```python
from build123d import *

# Parameters (mm, degrees)
F0_W     = 75
F0_H     = 75
F1_DEPTH = 75
F2_W     = 25
F2_H     = 25
F3_DEPTH = 25
F4_W     = 25
F4_H     = 25
F5_DEPTH = 25


with BuildPart() as f1:
    # F0 (on Top) → F1 (new body)
    with BuildSketch(Plane.XY):
        with Locations((-11.791817, -4.223716)):
            Rectangle(F0_W, F0_H)
    extrude(amount=F1_DEPTH)

    # F2 (on face) → F3 (cut)
    with BuildSketch(Plane(origin=(0, 0, 0), x_dir=(1, 0, 0), z_dir=(0, 0, -1))):
        with Locations((-36.791817, 29.223716)):
            Rectangle(F2_W, F2_H)
        with Locations((-36.791817, -20.776284)):
            Rectangle(F2_W, F2_H)
        with Locations((13.208183, 29.223716)):
            Rectangle(F2_W, F2_H)
        with Locations((13.208183, -20.776284)):
            Rectangle(F2_W, F2_H)
    extrude(amount=-F3_DEPTH, mode=Mode.SUBTRACT)

    # F4 (on face) → F5 (cut)
    with BuildSketch(Plane.XY.offset(75)):
        with Locations((-36.791817, 20.776284)):
            Rectangle(F4_W, F4_H)
        with Locations((13.208183, 20.776284)):
            Rectangle(F4_W, F4_H)
        with Locations((-36.791817, -29.223716)):
            Rectangle(F4_W, F4_H)
        with Locations((13.208183, -29.223716)):
            Rectangle(F4_W, F4_H)
    extrude(amount=-F5_DEPTH, mode=Mode.SUBTRACT)


solid = f1.part
```
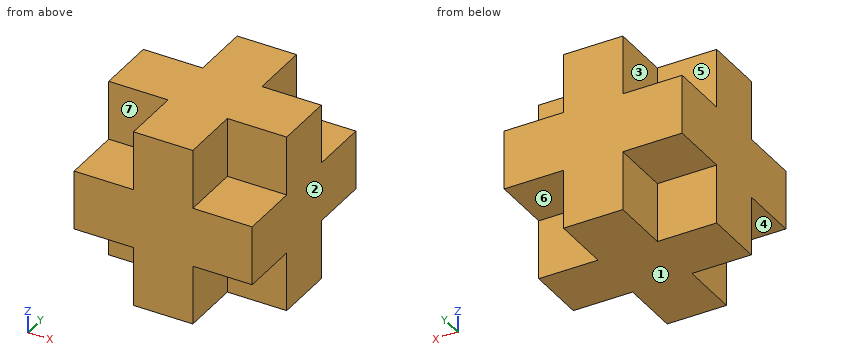
Verification items for the finished model (mm, model axes). Face numbers are marked on the shaded views. A direction names the side the tool comes from. Round coordinates to 2 decimals unless told otherwise and drop trailing zeros. Order: outer loops, then holes, each group sorted by start corner. A loop starts at its lowest first (then second) coordinate and runs counter-clockwise, first axis right, second up. Notation, with made-up numbers: (54.25, -32) -> (89.25, -32) arc R20 ccw to (89.25, 3) -> close; hole circle Ø3 at (16.25, 17). An arc over 180 degrees is marked (long way). Put each result on its own line as item: value. Start each with the question number.
(1) Section check B-B (y = 13). Enter the section's corners in (x, z).
(2) Draft check along X on the marked faces 1, 2 and 3. Enter one of: +X half, -X half, draft (parallel to the pull), parting line (faces both ways), or undercut.
(3) Tool access check on the marked faces 4, 5, 6 and 7. Record the directions out of +Z, -Z, +X, -X, +Y, -Y that give a thin tool (end or side, any length) a straight path to the whole face; none if there is none.
(4) Material ranges on line 1 along X through (y, z) = (-22.5, 68); line 2 along Y through (x, z) = (-38, 61); line 3 along Z through (x, y) = (-35.5, 17), recorded low to high.
(5) Depth check by flat-ended pin: pin 1 Ø12.5 at (y, z) = (-25.5, 15.5) entering from +X; pin 2 Ø20 at (x, z) = (-35.5, 66) entering from +Y; pin 3 Ø7.5 at (x, z) = (19, 68) entering from -Y; pin 4 Ø12 at (x, z) = (-28, 10.5) entering from -Y. Enter the tip coordinate at first touch or a pass-through.
(6) Section check A-A (x = 14). Enter the section's corners in (y, z).
Completed:
1. outline: (-49.29, 25) -> (-24.29, 25) -> (-24.29, 0) -> (0.71, 0) -> (0.71, 25) -> (25.71, 25) -> (25.71, 50) -> (0.71, 50) -> (0.71, 75) -> (-24.29, 75) -> (-24.29, 50) -> (-49.29, 50) -> close
2. face 1: draft
2. face 2: +X half
2. face 3: -X half
3. face 4: -Z, -X, -Y
3. face 5: +Z, -X, +Y
3. face 6: -Z, +X, +Y
3. face 7: +Z, -X, -Y
4. line 1: x = -24.29 to 0.71
4. line 2: y = -16.72 to 8.28
4. line 3: z = 25 to 50
5. pin 1: stops at x = 0.71
5. pin 2: stops at y = 8.28
5. pin 3: stops at y = -16.72
5. pin 4: stops at y = -41.72
6. outline: (-41.72, 25) -> (-16.72, 25) -> (-16.72, 0) -> (8.28, 0) -> (8.28, 25) -> (33.28, 25) -> (33.28, 50) -> (8.28, 50) -> (8.28, 75) -> (-16.72, 75) -> (-16.72, 50) -> (-41.72, 50) -> close
